The listing builds one solid part. Answer for the finished solid, in the listing's coordinates (mm). A direction names the side the tool comes from. Round coordinates to 2 decimals unless told otherwise and drop trailing zeros. Order: outer loops, then holes, each group sorted by start corner. A loop starts at its lowest first (then second) coordinate and runs counter-clockwise, first axis right, second up. Notation, with made-up numbers: M 87.25,63.25 L 95.25,63.25 A20 ccw 95.25,94.25 Z; hole C 64,-27 d4. An arc over 180 degrees is marked long. Put each result on its own line as item: value. Start each with the question number.
1. The part is cut by section B-B (z = 10). Give the vertices of the cut face in (x, y).
2. The mould has two halves that part along X. Classify faces 1 (the face through (2, 0, 2)), 2 (the face through (-11.05, 0.74, -1.83)), 3 (the face through (28, 1, 6)): +X half, -X half, draft (parallel to the pull), parting line (faces both ways), or undercut.
3. Which of the six approach directions +Z, -Z, +X, -X, +Y, -Y give full straight-line access (tool end or side, diameter ignored) to faces 4 (the face through (-7.82, 0.76, 10.82)), 5 (the face through (5, 1, -2)), 6 (the face through (11.55, 0.74, 16.08))?
4. The part is cut by section A-A (x = -7.5). Give the vertices of the cut face in (y, z).
5. Consider line 1 (X direction, y = 0.5, z = -2); line 2 (Z direction, x = 25, y = 1.1); line 3 (X direction, y = 0.7, z = 9.5). Determine where each line is inside the solid, lowest interval first.
6. The part is cut by section C-C (z = 6). Give the vertices of the cut face in (x, y).
7. Each of these flat-tipped pins is pushed along its axis until it touches: pin 1 Ø6 at (x, z) = (15, 20.5) entering from +Y; pin 2 Ø3 at (x, z) = (10, -1.5) entering from -Y; pin 3 Ø0.5 at (x, y) = (1, 1) entering from +Z. Where does it stop, or does it pass through?
Autodesk Inventor part; units mm, degrees
ref_plane "YZ Plane" through (0, 0, 0) normal (1, 0, 0) x (0, 1, 0)
ref_plane "XZ Plane" through (0, 0, 0) normal (0, 1, 0) x (-1, 0, 0)
ref_plane "XY Plane" through (0, 0, 0) normal (0, 0, 1) x (1, 0, 0)
sketch "スケッチ1" plane through (0, 0, 0) normal (0, 1, 0) x (-1, 0, 0)
  line L0 (5, 0) -> (-5, 0)
  line L1 (-5, 0) -> (-5, -3)
  line L2 (-5, -3) -> (5, -3)
  line L3 (5, -3) -> (5, 0)
  circle A0 centre (3.9, 0) radius 1.1
  line L4 (0, -3) -> (0, 0) construction
  circle A1 centre (-3.9, 0) radius 1.1
  line L5 (-5, -1.5) -> (5, -1.5) construction
  circle A2 centre (3.9, -3) radius 1.1
  circle A3 centre (-3.9, -3) radius 1.1
  circle A4 centre (-10, -1.5) radius 1.1
  circle A5 centre (10, -1.5) radius 1.1
  circle A6 centre (10, -1.5) radius 2
  circle A7 centre (-10, -1.5) radius 2
  line L6 (10, -3.5) -> (-10, -3.5)
  line L7 (-5, -3) -> (-5, -3.5)
  line L8 (5, -3) -> (5, -3.5)
  circle A8 centre (-25, 6) radius 1.6
  circle A9 centre (5, 21) radius 1.6
  line L9 (-25, 6) -> (5, 6) construction
  line L10 (5, 6) -> (5, 21) construction
  line L11 (5, 21) -> (-25, 6) construction
  circle A10 centre (-25, 6) radius 3
  circle A11 centre (5, 21) radius 3
  line L12 (11.9694, -1.1513) -> (7.954, 21.5231)
  line L13 (-10.7862, -3.339) -> (-26.1793, 3.2415)
  line L14 (-26.3416, 8.6833) -> (3.6584, 23.6833)
  point P0 (-2.8, 0)
  point P1 (2.8, 0)
  dimension "d2" = 2.2
  dimension "d0" = 10
  dimension "d1" = 3
  dimension "d3" = 2.2
  dimension "d4" = 5
  dimension "d5" = 4
  dimension "d6" = 4
  dimension "d7" = 3.2
  dimension "d8" = 3.2
  dimension "d9" = 15
  dimension "d10" = 30
  dimension "d11" = 6
  dimension "d12" = 6
  dimension "d15" = 15
  dimension "d17" = 6
extrude "押し出し1" add sketch "スケッチ1" along normal blind 1.5 contours A1 L1 L7 L6 A7 L13 A10 L14 A11 L12 A6 L8 L3 A0 L0 | A7 | A6 | A10 | A11
sketch "スケッチ2" plane through (0, 1.5, 0) normal (0, 1, 0) x (1, 0, 0)
  line L0 (-9.1854, -3.1) -> (-5.7511, -22.4936)
  line L1 (-5.7511, -22.4936) -> (27.378, -5.929)
  line L2 (27.378, -5.929) -> (20.7603, -3.1)
  line L3 (20.7603, -3.1) -> (-9.1854, -3.1)
  line L4 (10, 3.5) -> (5, 3.5)
  line L5 (26.1793, -3.2415) -> (10.7862, 3.339)
  line L6 (-11.9694, 1.1513) -> (-7.954, -21.5231)
  line L7 (-3.6584, -23.6833) -> (26.3416, -8.6833)
  arc A0 (2.8, 0) -> (5, 0) centre (3.9, 0) ccw
  line L8 (-3.6584, -23.6833) -> (26.3416, -8.6833)
  arc A1 (26.3416, -8.6833) -> (26.1793, -3.2415) centre (25, -6) ccw
  line L9 (26.1793, -3.2415) -> (10.7862, 3.339)
  arc A2 (10.7862, 3.339) -> (10, 3.5) centre (10, 1.5) ccw
  line L10 (10, 3.5) -> (5, 3.5)
  line L11 (5, 3.5) -> (5, 0)
  arc A3 (2.8, 0) -> (5, 0) centre (3.9, 0) ccw
  line L12 (2.8, 0) -> (-2.8, 0)
  arc A4 (-5, 0) -> (-2.8, 0) centre (-3.9, 0) ccw
  line L13 (-5, 0) -> (-5, 3.5)
  line L14 (-5, 3.5) -> (-10, 3.5)
  arc A5 (-10, 3.5) -> (-11.9694, 1.1513) centre (-10, 1.5) ccw
  line L15 (-11.9694, 1.1513) -> (-7.954, -21.5231)
  arc A6 (-7.954, -21.5231) -> (-3.6584, -23.6833) centre (-5, -21) ccw
  circle A7 centre (10, 1.5) radius 1.1
  circle A8 centre (25, -6) radius 1.6
  circle A9 centre (-10, 1.5) radius 1.1
  circle A10 centre (-5, -21) radius 1.6
  circle A11 centre (-5, -21) radius 3
  circle A12 centre (25, -6) radius 3
  point P0 (0, 0)
  point P1 (3.9, -1.1)
  point P2 (-6.4779, -18.3893)
  point P3 (-2.023, -20.6295)
  point P4 (22.9174, -8.1593)
  point P5 (22.7923, -3.9687)
  dimension "d18" = 2
  dimension "d19" = 2
  dimension "d20" = 2
  dimension "d22" = 2
extrude "押し出し2" cut sketch "スケッチ2" against normal through all contours L3 L2 A12 L1 A11 L0
fillet "フィレット1" radius 2 6 edges at (22.7923, 0.75, 3.9687) (22.9174, 0.75, 8.1593) (20.7603, 0.75, 3.1) (-9.1854, 0.75, 3.1) (-2.023, 0.75, 20.6295) (-6.4779, 0.75, 18.3893)
equation "\"d18\" = d22"
equation "\"d19\" = d18"
equation "\"d20\" = d19"
properties part number "momo" material "アルミニウム 2014-T4"
Resolved:
1. outline: M -9.99,0 L -7.96,0 L -7.96,1.5 L -9.99,1.5 Z; M 19.24,0 L 23.71,0 L 23.71,1.5 L 19.24,1.5 Z
2. face 1: draft
2. face 2: undercut
2. face 3: +X half
3. face 4: +Y, -Y
3. face 5: -Z, +Y, -Y
3. face 6: +Z, +X, +Y, -Y
4. outline: M 0,-3.5 L 1.5,-3.5 L 1.5,3.23 L 0,3.23 Z; M 0,12.62 L 1.5,12.62 L 1.5,22.66 L 0,22.66 Z
5. line 1: -11.94 to -10.98, -9.02 to -5, 5 to 9.02, 10.98 to 13.92
5. line 2: 2.74 to 4.4, 7.6 to 9.35
5. line 3: -10.08 to -8.05, 20.24 to 24.71
6. outline: M -10.7,0 L -8.67,0 L -8.67,1.5 L -10.7,1.5 Z; M 22,0 L 23.4,0 L 23.4,1.5 L 22,1.5 Z; M 26.6,0 L 28,0 L 28,1.5 L 26.6,1.5 Z
7. pin 1: through
7. pin 2: y = 0
7. pin 3: z = 21.48
